Geometry check sheet. Reference: the model listing, model coordinates, mm. Round coordinates to 2 decimals unless told otherwise and drop trailing zeros. Write each loop counter-clockwise with the first axis right and the second up, starting at its lowest first coordinate (ties: lowest second). Pieces come first, ordered by that corner, then holes.
Item 1: Cross-section at C-C (y = 19). Enter the section's corners in (x, z).
Item 2: Scan lines: probe 1 along Z at (x, y) = (17.5, 7); probe 2 along X at (y, z) = (18, 1); probe 3 along X at (y, z) = (16, 1.5). Record each from-to range of solid material in increasing order.
Item 3: Cross-section at A-A (z = 0.75). State how many separate pieces and enclosed holes the cut face has, then the cut area to 3 significant figures.
Item 4: Depth check by flat-ended pin: P1, Ø0.8, axis at y = 2.5, z = -0.5, coming from the +X side; P2, Ø5, axis at x = 21, y = 12.5, coming from the +Z side; P3, Ø1.1, axis at x = 28, y = 16.8, coming from the +Z side; P4, Ø0.5, axis at y = 2.5, z = -0.5, coming from the -X side. Enter the tip coordinate at first touch or a pass-through.
Item 5: Cross-section at D-D (y = 14.6). Enter the section's corners in (x, z).
Item 6: Cross-section at B-B (x = 28). Enter the section's corners in (y, z), then the cut area to 3 significant figures.
from build123d import *

# Parameters (mm, degrees)
PAD_DEPTH              = 2
SKETCH001_R            = 0.6
HOLE_DEPTH             = 2.001
LINEARPATTERN_COUNT    = 6
LINEARPATTERN_PITCH    = 2.2
POCKET_DEPTH           = 2.001
SKETCH003_W            = 20
SKETCH003_H            = 2
PAD001_DEPTH           = 5
SKETCH004_W            = 1
SKETCH004_H            = 1
REVOLUTION_ANGLE       = -90
LINEARPATTERN001_COUNT = 10
LINEARPATTERN001_PITCH = 1.888889
CHAMFER_SIZE           = 1.8
CHAMFER001_SIZE        = 2
CHAMFER002_SIZE        = 0.3


with BuildPart() as part:
    # Sketch → Pad (new body)
    with BuildSketch(Plane.XY):
        Polygon((0, 0), (20, 0), (20, 6), (30, 6), (30, 21), (20, 21), (0, 10), align=None)
    extrude(amount=PAD_DEPTH)

    # Sketch001 (on Face9 of Pad) → Hole (cut, through all)
    with BuildSketch(Plane.XY.offset(2)):
        with Locations((28, 19)):
            Circle(SKETCH001_R)
    hole = extrude(amount=-HOLE_DEPTH, mode=Mode.SUBTRACT)

    # LinearPattern: Hole ×6
    with Locations(*[(0, -i * LINEARPATTERN_PITCH, 0) for i in range(1, LINEARPATTERN_COUNT)]):
        add(hole, mode=Mode.SUBTRACT)

    # Sketch002 (on Face5 of LinearPattern) → Pocket (cut, through all)
    with BuildSketch(Plane.XY.offset(2)):
        Polygon((11.837454, 13.403028), (7.563314, 6), (16.111595, 6), align=None)
        Polygon((22.577143, 9.579128), (22.577143, 18.127408), (15.174115, 13.853268), align=None)
    extrude(amount=-POCKET_DEPTH, mode=Mode.SUBTRACT)

    # Sketch003 (on Face4 of Pocket) → Pad001 (join)
    with BuildSketch(Plane(origin=(0, 0, 0), x_dir=(1, 0, 0), z_dir=(0, 0, -1))):
        with Locations((10, -1)):
            Rectangle(SKETCH003_W, SKETCH003_H)
    extrude(amount=PAD001_DEPTH)

    # Sketch004 (on Face19 of Pad001) → Revolution (revolve)
    with BuildSketch(Plane(origin=(0, 2, 0), x_dir=(-1, 0, 0), z_dir=(0, 1, 0))):
        with Locations((-18.5, -0.5)):
            Rectangle(SKETCH004_W, SKETCH004_H)
    revolution = revolve(axis=Axis((10, 2, 0), (-1, 0, 0)), revolution_arc=REVOLUTION_ANGLE)

    # LinearPattern001: Revolution ×10
    with Locations(*[(-i * LINEARPATTERN001_PITCH, 0, 0) for i in range(1, LINEARPATTERN001_COUNT)]):
        add(revolution)

    # Chamfer
    chamfer_edges = [part.edges().sort_by_distance(p)[0] for p in [
        (10, 2, -5),
    ]]
    chamfer(chamfer_edges, length=CHAMFER_SIZE)

    # Chamfer001
    chamfer001_edges = [part.edges().sort_by_distance(p)[0] for p in [
        (10, 2, -3.2),
    ]]
    chamfer(chamfer001_edges, length=CHAMFER001_SIZE)

    # Chamfer002
    chamfer002_edges = [part.edges().sort_by_distance(p)[0] for p in [
        (10, 0.585786, -4.614214),
    ]]
    chamfer(chamfer002_edges, length=CHAMFER002_SIZE)


solid = part.part
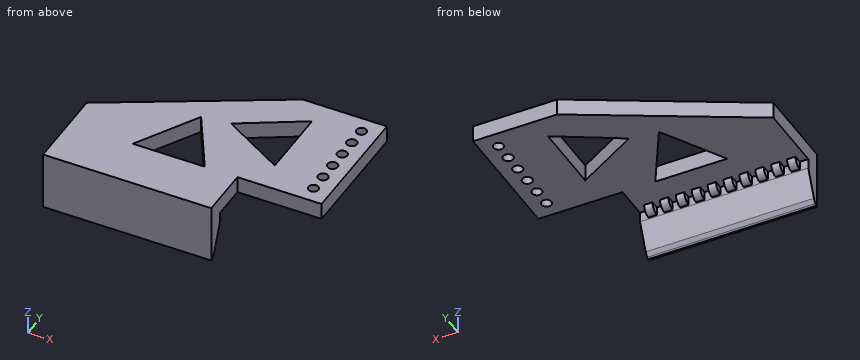
Resolved:
1. outline: (16.36, 0) - (27.4, 0) - (27.4, 2) - (16.36, 2) - close; (28.6, 0) - (30, 0) - (30, 2) - (28.6, 2) - close
2. probe 1: z = 0 to 2
2. probe 2: x = 14.55 to 22.36, 22.58 to 30
2. probe 3: x = 10.91 to 18.89, 22.58 to 30
3. separate pieces: 1
3. enclosed holes: 8
3. area: 390 mm2
4. P1: stops at x = 19
4. P2: stops at z = 2
4. P3: passes through
4. P4: stops at x = 1
5. outline: (8.36, 0) - (16.47, 0) - (16.47, 2) - (8.36, 2) - close; (22.58, 0) - (27.4, 0) - (27.4, 2) - (22.58, 2) - close; (28.6, 0) - (30, 0) - (30, 2) - (28.6, 2) - close
6. outline: (6, 0) - (7.4, 0) - (7.4, 2) - (6, 2) - close; (8.6, 0) - (9.6, 0) - (9.6, 2) - (8.6, 2) - close; (10.8, 0) - (11.8, 0) - (11.8, 2) - (10.8, 2) - close; (13, 0) - (14, 0) - (14, 2) - (13, 2) - close; (15.2, 0) - (16.2, 0) - (16.2, 2) - (15.2, 2) - close; (17.4, 0) - (18.4, 0) - (18.4, 2) - (17.4, 2) - close; (19.6, 0) - (21, 0) - (21, 2) - (19.6, 2) - close
6. area: 15.6 mm2
